Check sheet for the modelled part. Datum: model origin and axes. Units: mm. Face numbers are marked on the shaded views. A direction names the side the tool comes from. Round coordinates to 2 decimals unless told otherwise and drop trailing zeros. Write each loop counter-clockwise with the first axis right and the second up, starting at its lowest first coordinate (ties: lowest second). Pieces come first, ordered by that corner, then holes.
Item 1: Cross-section at A-A on z = 93. Enter the section's corners in (x, y).
Item 2: Material ranges on line 1 (Z direction, x = 49, y = 36); line 2 (X direction, y = 170, z = 233.5); line 3 (Z direction, x = 282.5, y = 252.5), recorded low to high.
Item 3: Cross-section at D-D on z = 683. Enter the section's corners in (x, y).
Item 4: Tool access check on the marked faces 1, 2, 3, 4 and 5. Record the directions out of +Z, -Z, +X, -X, +Y, -Y that give a thin tool (end or side, any length) a straight path to the whole face; none if there is none.
Item 5: Go/stop test with flat-tipped pins: pin 1 Ø1.5 at (x, y) = (81.5, 312) entering from +Z; pin 2 Ø21 at (y, z) = (337, 468.5) entering from -X; pin 3 Ø10 at (x, y) = (506, 267) entering from +Z. Record where each tip stops, or that it passes through.
Item 6: Cross-section at B-B on y = 258.5. Enter the section's corners in (x, z).
Item 7: Cross-section at C-C on z = 235. Enter the section's corners in (x, y), plus the area to 3 significant figures.
Item 8: Release check for a two-part mould opening along Z. For the marked faces 6, 7 and 8 record: +Z half, -Z half, draft (parallel to the pull), parting line (faces both ways), or undercut.
from build123d import *

# Parameters (mm, degrees)
F0_W      = 12
F0_H      = 358
F0_W_2    = 18
F0_H_2    = 18
F0_W_3    = 170
F0_H_3    = 12
F0_W_4    = 376
F0_H_4    = 182
F1_DEPTH  = 12
F2_DEPTH  = 250
F3_W      = 90
F3_H      = 210
F4_DEPTH  = 206.001
F5_W      = 90
F5_H      = 210
F6_DEPTH  = 25
F7_W      = 600
F7_H      = 400
F8_DEPTH  = 12
F11_DEPTH = 400
F12_W     = 90
F12_H     = 200
F12_H_2   = 210
F13_DEPTH = 20
F9_W      = 30
F9_H      = 30
F14_DEPTH = 250
F15_DEPTH = 250
F17_DEPTH = 130
F19_DEPTH = 160


with BuildPart() as f1:
    # F0 (on Top) → F1 (new body)
    with BuildSketch(Plane.XY):
        with Locations((6, 209)):
            Rectangle(F0_W, F0_H)
        Polygon((0, 400), (0, 388), (12, 388), (200, 388), (200, 400), align=None)
        Polygon((30, 30), (30, 12), (200, 12), (200, 388), (12, 388), (12, 30), align=None)
        Polygon((0, 30), (0, 0), (30, 0), (30, 12), (12, 12), (12, 30), align=None)
        with Locations((21, 21)):
            Rectangle(F0_W_2, F0_H_2)
        with Locations((115, 6)):
            Rectangle(F0_W_3, F0_H_3)
        Polygon((200, 388), (200, 12), (212, 12), (212, 194), (212, 206), (212, 388), align=None)
        with Locations((206, 6)):
            Rectangle(F0_W, F0_H_3)
        with Locations((400, 6)):
            Rectangle(F0_W_4, F0_H_3)
        with Locations((400, 103)):
            Rectangle(F0_W_4, F0_H_4)
        with Locations((400, 200)):
            Rectangle(F0_W_4, F0_H_3)
        with Locations((400, 297)):
            Rectangle(F0_W_4, F0_H_4)
        with Locations((400, 394)):
            Rectangle(F0_W_4, F0_H_3)
        with Locations((594, 200)):
            Rectangle(F0_W, F0_H_3)
        with Locations((206, 394)):
            Rectangle(F0_W, F0_H_3)
        Polygon((588, 400), (588, 388), (588, 206), (600, 206), (600, 400), align=None)
        Polygon((588, 12), (588, 0), (600, 0), (600, 194), (588, 194), align=None)
    extrude(amount=-F1_DEPTH)

    # F0 (on Top) → F2 (join)
    with BuildSketch(Plane.XY):
        Polygon((0, 400), (0, 388), (12, 388), (200, 388), (200, 400), align=None)
        with Locations((206, 394)):
            Rectangle(F0_W, F0_H_3)
        Polygon((200, 388), (200, 12), (212, 12), (212, 194), (212, 206), (212, 388), align=None)
        with Locations((206, 6)):
            Rectangle(F0_W, F0_H_3)
        with Locations((21, 21)):
            Rectangle(F0_W_2, F0_H_2)
        Polygon((0, 30), (0, 0), (30, 0), (30, 12), (12, 12), (12, 30), align=None)
        with Locations((400, 200)):
            Rectangle(F0_W_4, F0_H_3)
        with Locations((594, 200)):
            Rectangle(F0_W, F0_H_3)
        Polygon((588, 400), (588, 388), (588, 206), (600, 206), (600, 400), align=None)
        Polygon((588, 12), (588, 0), (600, 0), (600, 194), (588, 194), align=None)
    extrude(amount=F2_DEPTH)

    # F3 (on face) → F4 (cut, through all)
    with BuildSketch(Plane.XZ.offset(-194)):
        with Locations((297, 105)):
            Rectangle(F3_W, F3_H)
    extrude(amount=-F4_DEPTH, mode=Mode.SUBTRACT)

    # F5 (on face) → F6 (cut)
    with BuildSketch(Plane(origin=(200, 0, 0), x_dir=(0, -1, 0), z_dir=(-1, 0, 0))):
        with Locations((-85, 105)):
            Rectangle(F5_W, F5_H)
    extrude(amount=-F6_DEPTH, mode=Mode.SUBTRACT)

    # F7 (on face) → F8 (join)
    with BuildSketch(Plane.XY.offset(250)):
        with Locations((300, 200)):
            Rectangle(F7_W, F7_H)
    extrude(amount=F8_DEPTH)

    # F10 (on face) → F11 (join)
    with BuildSketch(Plane.XZ):
        Polygon((0, 524), (0, 512), (12, 512), (200, 512), (200, 262), (212, 262), (212, 524), (212, 739), (588, 612), (588, 262), (600, 262), (600, 620.6128402984), (200, 755.7192232772), (200, 524), align=None)
    extrude(amount=-F11_DEPTH)

    # F12 (on face) → F13 (cut)
    with BuildSketch(Plane(origin=(200, 0, 0), x_dir=(0, -1, 0), z_dir=(-1, 0, 0))):
        with Locations((-317.7582192421, 624)):
            Rectangle(F12_W, F12_H)
        with Locations((-85, 367)):
            Rectangle(F12_W, F12_H_2)
    extrude(amount=-F13_DEPTH, mode=Mode.SUBTRACT)

    # F9 (on face) → F14 (join)
    with BuildSketch(Plane.XY.offset(262)):
        with Locations((15, 15)):
            Rectangle(F9_W, F9_H)
    extrude(amount=F14_DEPTH)

    # F9 (on face) → F15 (join)
    with BuildSketch(Plane.XY.offset(262)):
        Polygon((212, 400), (0, 400), (0, 388), (200, 388), (212, 388), align=None)
    extrude(amount=F15_DEPTH)

    # F16 (on face) → F17 (join)
    with BuildSketch(Plane(origin=(0, 400, 0), x_dir=(-1, 0, 0), z_dir=(0, 1, 0))):
        Polygon((-212, 262), (-212, 524), (-238, 524), (-238, 497.8), (-264, 497.8), (-264, 471.6), (-290, 471.6), (-290, 445.4), (-316, 445.4), (-316, 419.2), (-342, 419.2), (-342, 393), (-368, 393), (-368, 366.8), (-394, 366.8), (-394, 340.6), (-420, 340.6), (-420, 314.4), (-446, 314.4), (-446, 288.2), (-472, 288.2), (-472, 262), align=None)
    extrude(amount=-F17_DEPTH)

    # F18 (on face) → F19 (cut)
    with BuildSketch(Plane.XZ.offset(-270)):
        Polygon((212, 262), (460, 262), (460, 276.2), (434, 276.2), (434, 302.4), (408, 302.4), (408, 328.6), (382, 328.6), (382, 354.8), (356, 354.8), (356, 381), (330, 381), (330, 407.2), (304, 407.2), (304, 433.4), (278, 433.4), (278, 459.6), (252, 459.6), (252, 485.8), (226, 485.8), (226, 512), (212, 512), align=None)
    extrude(amount=-F19_DEPTH, mode=Mode.SUBTRACT)


solid = f1.part
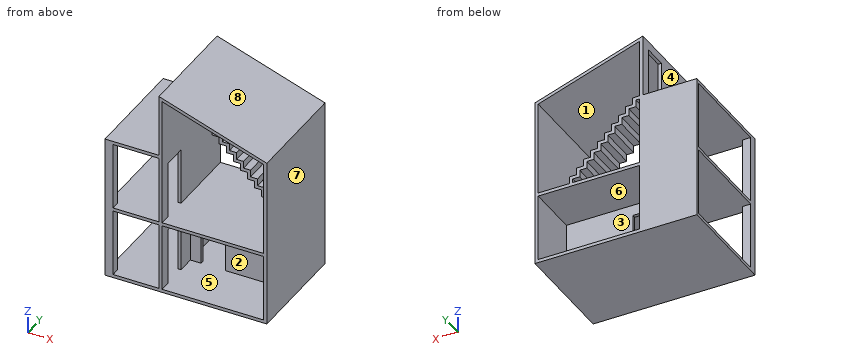
Response values:
1. outline: (0, 0) - (30, 0) - (30, 30) - (0, 30) - close; (0, 388) - (200, 388) - (200, 130) - (212, 130) - (212, 194) - (252, 194) - (252, 206) - (212, 206) - (212, 400) - (0, 400) - close; (200, 0) - (212, 0) - (212, 40) - (200, 40) - close; (342, 194) - (588, 194) - (588, 0) - (600, 0) - (600, 400) - (588, 400) - (588, 206) - (342, 206) - close
2. line 1: z = -12 to 0, 250 to 262, 512 to 524
2. line 2: x = 200 to 212, 588 to 600
2. line 3: z = -12 to 0, 250 to 262, 715.19 to 727.85
3. outline: (200, 0) - (212, 0) - (212, 272.76) - (200, 272.76) - close; (200, 362.76) - (212, 362.76) - (212, 400) - (200, 400) - close; (377.8, 0) - (415.29, 0) - (415.29, 400) - (377.8, 400) - close
4. face 1: +Y, -Y
4. face 2: -Y
4. face 3: +Y
4. face 4: +Z, -X, +Y, -Y
4. face 5: none
5. pin 1: stops at z = 524
5. pin 2: stops at x = 200
5. pin 3: stops at z = 654.05
6. outline: (0, -12) - (600, -12) - (600, 620.61) - (200, 755.72) - (200, 524) - (0, 524) - (0, 512) - (200, 512) - (200, 262) - (0, 262) - (0, 250) - (200, 250) - (200, 0) - (0, 0) - close; hole (212, 0) - (588, 0) - (588, 250) - (212, 250) - close; hole (212, 262) - (588, 262) - (588, 612) - (212, 739) - close
7. outline: (0, 0) - (30, 0) - (30, 30) - (0, 30) - close; (0, 388) - (200, 388) - (200, 0) - (212, 0) - (212, 194) - (588, 194) - (588, 0) - (600, 0) - (600, 400) - (588, 400) - (588, 206) - (212, 206) - (212, 400) - (0, 400) - close
7. area: 17,400 mm2
8. face 6: undercut
8. face 7: draft
8. face 8: +Z half
